Could you check a few things on this model? Use its own coordinates, in mm. A direction names the side the tool comes from. Give positions to 0.01 mm unless a question says otherwise; leave off trailing zeros. Loops run counter-clockwise (first coordinate to the right, second up) from the corner with the lowest first, then second, coordinate; pieces in that order, holes last. Notation, with made-up numbers: M 12,68.5 L 50,68.5 A19 cw 50,72.5 Z; hole C 14.5,76 d7. An arc over 180 degrees is marked long. Answer in a Markdown table with one row per item. Add a question column.
1. Which directions (+Z, -Z, +X, -X, +Y, -Y) give clear straight access to the entire face, cutting with the end or side of a thin tool? Please do faces 1 (the cylindrical face through (65.215, 3.757, 8.234)), 2 (the flat face through (149, 3, 9)), 3 (the flat face through (23, 6, 10)).
2. If we section it at A-A on x = 67: List the corners of the cut face in (y, z) for me, then the cut area to 3 significant figures.
3. If we section it at C-C on z = -8.5: List the corners of the cut face in (x, y) for me.
4. Thinking about a two-plate mould opening in X: for faces 4 (the flat face through (17, 3, 9)), 5 (the flat face through (88, 9.5, 2)), 6 (the cylindrical face through (156.757, 3.757, 8.39)), which applies, released by +X, released by -X, zero draft, split by the parting line, or undercut?
5. I'm going to push flat-ended pins straight in: pin 1 Ø3 at (x, z) = (133, -3) entering from +Y; pin 2 Ø6 at (x, z) = (155, 8) entering from -Y; pin 3 Ø3 at (x, z) = (120, -7) entering from -Y; pin 4 Ø9 at (x, z) = (157, 7.5) entering from +Y. Where does each tip first touch, or does it pass through?
6. If we section it at B-B on z = 8: Count the separate pieces of the cut face and the enclosed holes in it, then the cut area to 3 significant figures.
7. I need wall thicknesses on line 1 along Y through (x, z) = (150.5, 3.5); line 2 along Z through (x, y) = (155, 4.95); line 3 along Z through (x, y) = (67, 3.4). Which ranges of each line are inside material? Lowest first, please. Write a range as from..to.
Autodesk Inventor part; units mm, degrees
ref_plane "YZ Plane" through (0, 0, 0) normal (1, 0, 0) x (0, 1, 0)
ref_plane "XZ Plane" through (0, 0, 0) normal (0, 1, 0) x (-1, 0, 0)
ref_plane "XY Plane" through (0, 0, 0) normal (0, 0, 1) x (1, 0, 0)
sketch "Sketch3" plane through (0, 0, 0) normal (1, 0, 0) x (0, 1, 0)
  line L0 (0, 0) -> (10, 0)
  line L1 (10, 0) -> (10, -10)
  line L2 (10, -10) -> (0, -10)
  line L3 (0, -10) -> (0, 0)
  line L4 (10, 0) -> (0, -10)
  line L5 (6, 0) -> (0, 0)
  line L6 (0, 0) -> (0, 12)
  line L7 (0, 12) -> (6, 12)
  line L8 (6, 12) -> (6, 0)
  line L9 (9.5, 0) -> (6, 0)
  line L10 (6, 0) -> (6, 4)
  line L11 (6, 4) -> (9.5, 4)
  line L12 (9.5, 4) -> (9.5, 0)
  dimension "d30" = 12
  dimension "d31" = 6
  dimension "d63" = 10
  dimension "d74" = 0.5
  dimension "d75" = 4
  dimension "d76" = 3.5
  dimension "d141" = 45
  dimension "d142" = 10
extrude "Extrusion2" add sketch "Sketch3" along normal blind 178 contours L6 L7 L8 L0 | L0 L4 L3 | L8 L11 L12 L0
sketch "Sketch10" plane through (0, 0, -10) normal (0, -1, 0) x (1, 0, 0)
  line L0 (0, 14) -> (0, 22)
  line L1 (0, 22) -> (178, 22)
  line L2 (178, 14) -> (178, 22)
  line L3 (0, 14) -> (178, 14)
  line L4 (0, 10) -> (0, 14)
  line L5 (0, 14) -> (17, 14)
  line L6 (17, 14) -> (17, 22)
  line L7 (17, 22) -> (0, 22)
  line L8 (0, 22) -> (0, 14)
  line L9 (0, 14) -> (178, 14)
  line L10 (178, 22) -> (161, 22)
  line L11 (161, 22) -> (161, 14)
  line L12 (161, 14) -> (178, 14)
  line L13 (178, 14) -> (178, 22)
  line L14 (17, 22) -> (29, 22)
  line L15 (29, 22) -> (29, 14)
  line L16 (29, 14) -> (17, 14)
  line L17 (17, 14) -> (17, 22)
  line L18 (61, 22) -> (73, 22)
  line L19 (73, 22) -> (73, 14)
  line L20 (73, 14) -> (61, 14)
  line L21 (61, 14) -> (61, 22)
  line L22 (105, 22) -> (117, 22)
  line L23 (117, 22) -> (117, 14)
  line L24 (117, 14) -> (105, 14)
  line L25 (105, 14) -> (105, 22)
  line L26 (149, 22) -> (161, 22)
  line L27 (161, 22) -> (161, 14)
  line L28 (161, 14) -> (149, 14)
  line L29 (149, 14) -> (149, 22)
  line L30 (17, 22) -> (29, 14)
  line L31 (29, 22) -> (17, 14)
  line L32 (61, 22) -> (73, 14)
  line L33 (73, 22) -> (61, 14)
  line L34 (105, 22) -> (117, 14)
  line L35 (117, 22) -> (105, 14)
  line L36 (149, 22) -> (161, 14)
  line L37 (161, 22) -> (149, 14)
  point P0 (105, 14)
  point P1 (23, 18)
  point P2 (67, 18)
  point P3 (111, 18)
  point P4 (155, 18)
  dimension "d118" = 17
  dimension "d119" = 17
  dimension "d120" = 12
  dimension "d121" = 12
  dimension "d122" = 12
  dimension "d123" = 12
  dimension "d124" = 0
  dimension "d125" = 0
  dimension "d126" = 32
  dimension "d129" = 32
  dimension "d130" = 32
extrude "Extrusion5" cut sketch "Sketch10" against normal up to next contours L0 L1 L6 L3 | L15 L1 L21 L3 | L19 L1 L25 L3 | L23 L1 L29 L3 | L11 L1 L2 L3
hole "Hole4" at (23, 0, 8) at (67, 0, 8) at (111, 0, 8) at (155, 0, 8) direction (0, 1, 0) diameter 3.6 end through all countersink diameter 6.5 countersink angle 90
fillet "Fillet2" radius 2 8 edges at (17, 3, 4) (29, 3, 4) (61, 3, 4) (73, 3, 4) (105, 3, 4) (117, 3, 4) (149, 3, 4) (161, 3, 4)
equation "\"d126\" = d130"
equation "\"d129\" = d130"
properties part number "plog" material "Steel, Alloy"
Results:
| question | item | result |
|---|---|---|
| 1 | face 1 | +Y, -Y |
| 1 | face 2 | +Z, +Y, -Y |
| 1 | face 3 | +Z, +X, -X, +Y |
| 2 | outline | M 0,-10 L 10,0 L 9.5,0 L 9.5,4 L 6,4 L 6,6.2 L 1.45,6.2 L 0,4.75 Z; M 0,11.25 L 1.45,9.8 L 6,9.8 L 6,12 L 0,12 Z |
| 2 | area | 112 mm2 |
| 3 | outline | M 0,0 L 178,0 L 178,1.5 L 0,1.5 Z |
| 4 | face 4 | released by -X |
| 4 | face 5 | zero draft |
| 4 | face 6 | undercut |
| 5 | pin 1 | y = 8.5 |
| 5 | pin 2 | y = 0.25 |
| 5 | pin 3 | y = 0 |
| 5 | pin 4 | y = 9.5 |
| 6 | separate pieces | 8 |
| 6 | enclosed holes | 0 |
| 6 | area | 193 mm2 |
| 7 | line 1 | 0..9.5 |
| 7 | line 2 | -5.05..6.2, 9.8..12 |
| 7 | line 3 | -6.6..6.2, 9.8..12 |
